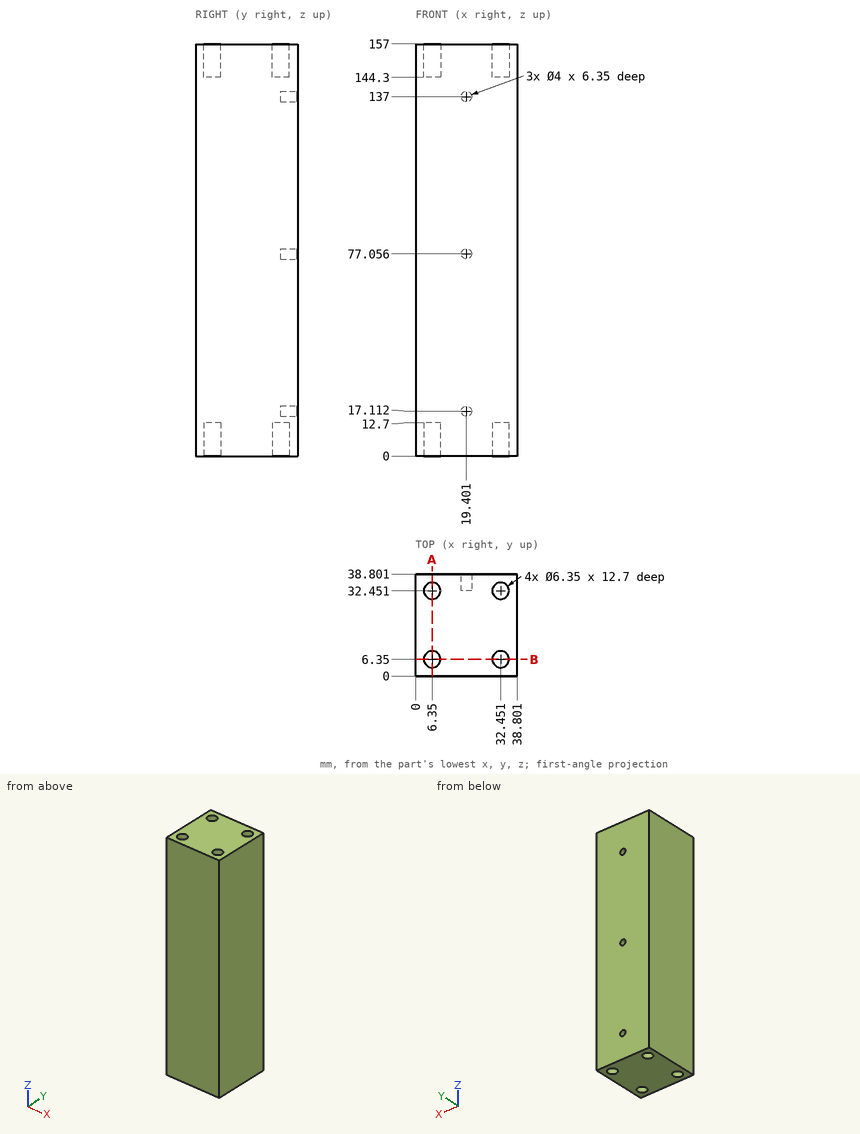
Geometry: see drawing. Coordinates: mm, zero at the bounding-box minimum. Round coordinates to 2 decimals unless told otherwise and drop trailing zeros. Write each loop counter-clockwise with the first axis right and the second up, starting at its lowest first coordinate (ties: lowest second). Pieces come first, ordered by that corner, then holes.
Item 1: Pin query (flat end, axial travel): P1, Ø8, axis at y = 15.5, z = 110.5, coming from the -X side; P2, Ø1.2, axis at x = 19.5, z = 17, coming from the +Y side; P3, Ø5, axis at x = 6.35, y = 32.45, coming from the -Z side. Return the tip coordinate at first contact, or that it passes through.
Item 2: Section query A-A (x = 6.35). Return loops of the section in (y, z) (1 decimal).
Item 3: Material intervals for L1, parallel to X at y = 6, z = 6 (1 decimal); L2, parallel to Z at x = 5, y = 5, sorted ascending.
Completed:
1. P1: stops at x = 0
1. P2: stops at y = 32.45
1. P3: stops at z = 12.7
2. outline: (0, 0) - (3.2, 0) - (3.2, 12.7) - (9.5, 12.7) - (9.5, 0) - (29.3, 0) - (29.3, 12.7) - (35.6, 12.7) - (35.6, 0) - (38.8, 0) - (38.8, 157) - (35.6, 157) - (35.6, 144.3) - (29.3, 144.3) - (29.3, 157) - (9.5, 157) - (9.5, 144.3) - (3.2, 144.3) - (3.2, 157) - (0, 157) - close
3. L1: x = 0 to 3.2, 9.5 to 29.3, 35.6 to 38.8
3. L2: z = 12.7 to 144.3
